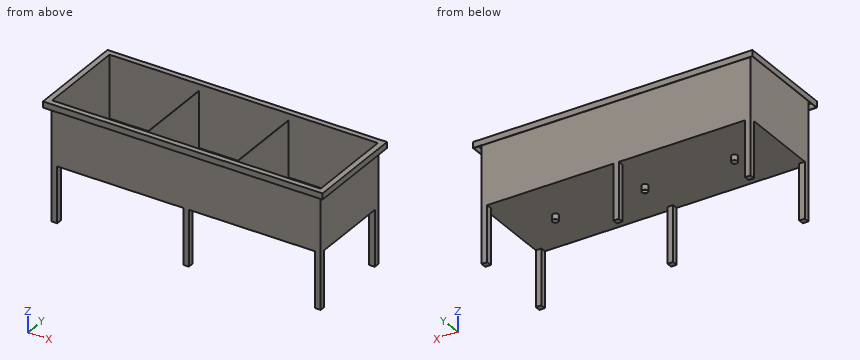
from build123d import *

# Parameters (mm, degrees)
F0_W      = 2412
F0_H      = 806
F1_DEPTH  = 563
F2_T      = -3
F3_W      = 3
F3_H      = 800
F4_DEPTH  = 500
F5_W      = 2506
F5_H      = 900
F5_W_2    = 2412
F5_H_2    = 806
F6_DEPTH  = 4
F7_R      = 25
F8_DEPTH  = 25
F9_R      = 27
F9_R_2    = 25
F10_DEPTH = 50
F11_W     = 2506
F11_H     = 900
F11_W_2   = 2500
F11_H_2   = 894
F12_DEPTH = 50
F13_W     = 50
F13_H     = 50
F14_DEPTH = 500


with BuildPart() as f1:
    # F0 (on Top) → F1 (new body)
    with BuildSketch(Plane.XY):
        with Locations((-1206, -403)):
            Rectangle(F0_W, F0_H)
    extrude(amount=-F1_DEPTH)

    # F2
    f2_openings = [f1.faces().sort_by_distance(p)[0] for p in [
        (-1206, -403, 0),
    ]]
    offset(amount=F2_T, openings=f2_openings)

    # F3 (on face) → F4 (join)
    with BuildSketch(Plane.XY.offset(-560)):
        with Locations((-1607.5, -403)):
            Rectangle(F3_W, F3_H)
        with Locations((-804.5, -403)):
            Rectangle(F3_W, F3_H)
    extrude(amount=F4_DEPTH)

    # F5 (on face) → F6 (join)
    with BuildSketch(Plane.XY):
        with Locations((-1206, -403)):
            Rectangle(F5_W, F5_H)
        with Locations((-1206, -403)):
            Rectangle(F5_W_2, F5_H_2, mode=Mode.SUBTRACT)
    extrude(amount=-F6_DEPTH)

    # F7 (on face) → F8 (cut)
    with BuildSketch(Plane.XY.offset(-560)):
        with Locations((-2009, -403)):
            Circle(F7_R)
        with Locations((-1206, -403)):
            Circle(F7_R)
        with Locations((-403, -403)):
            Circle(F7_R)
    extrude(amount=-F8_DEPTH, mode=Mode.SUBTRACT)

    # F9 (on face) → F10 (join)
    with BuildSketch(Plane(origin=(0, 0, -563), x_dir=(1, 0, 0), z_dir=(0, 0, -1))):
        with Locations((-1206, 403)):
            Circle(F9_R)
        with Locations((-1206, 403)):
            Circle(F9_R_2, mode=Mode.SUBTRACT)
        with Locations((-2009, 403)):
            Circle(F9_R)
        with Locations((-2009, 403)):
            Circle(F9_R_2, mode=Mode.SUBTRACT)
        with Locations((-403, 403)):
            Circle(F9_R)
        with Locations((-403, 403)):
            Circle(F9_R_2, mode=Mode.SUBTRACT)
    extrude(amount=F10_DEPTH)

    # F11 (on face) → F12 (join)
    with BuildSketch(Plane(origin=(0, 0, -4), x_dir=(1, 0, 0), z_dir=(0, 0, -1))):
        with Locations((-1206, 403)):
            Rectangle(F11_W, F11_H)
        with Locations((-1206, 403)):
            Rectangle(F11_W_2, F11_H_2, mode=Mode.SUBTRACT)
    extrude(amount=F12_DEPTH)

    # F13 (on face) → F14 (join)
    with BuildSketch(Plane(origin=(0, 0, -563), x_dir=(1, 0, 0), z_dir=(0, 0, -1))):
        with Locations((-2387, 781)):
            Rectangle(F13_W, F13_H)
        with Locations((-2387, 25)):
            Rectangle(F13_W, F13_H)
        with Locations((-25, 781)):
            Rectangle(F13_W, F13_H)
        with Locations((-25, 25)):
            Rectangle(F13_W, F13_H)
        with Locations((-1206, 781)):
            Rectangle(F13_W, F13_H)
        with Locations((-1206, 25)):
            Rectangle(F13_W, F13_H)
    extrude(amount=F14_DEPTH)


solid = f1.part
Verification items for the finished model (mm, model axes). Give positions to 0.01 mm unless a question says otherwise; leave off trailing zeros. Order: outer loops, then holes, each group sorted by start corner. A loop starts at its lowest first (then second) coordinate and runs counter-clockwise, first axis right, second up. Notation, with made-up numbers: M -28,41 L -23,41 A32 ccw -23,67 Z; hole C 12,82 d5. An arc over 180 degrees is marked long. Answer as a JSON object with one key per item and string values. Group by question number.
1) Cross-section at D-D (x = -611). Enter the section's corners in (y, z), then the cut area to 3 significant figures.
2) Cross-section at A-A (x = -2009). Enter the section's corners in (y, z).
3) Cross-section at B-B (z = -742). Enter the section's corners in (x, y), then the cut area to 3 significant figures.
4) Cross-section at C-C (y = -180.5). Enter the section's corners in (x, z).
5) Scan lines: line 1 along Y through (x, z) = (-1206, -598); line 2 along X through (y, z) = (-475.5, -450.5); line 3 along X through (y, z) = (-403, -595.5). Record each from-to range of solid material in increasing order. Write a range as [from, to].
6) Depth check by flat-ended pin: pin 1 Ø8 at (x, z) = (-1311, -336) entering from +Y; pin 2 Ø25 at (y, z) = (-774.5, -838.5) entering from -X; pin 3 Ø3 at (y, z) = (-69, -460) entering from +X. Enter the tip coordinate at first touch or a pass-through.
Result sheet:
{
 "1": {"outline": "M -853,-54 L -850,-54 L -850,-4 L -806,-4 L -806,-563 L 0,-563 L 0,-4 L 44,-4 L 44,-54 L 47,-54 L 47,0 L -3,0 L -3,-560 L -803,-560 L -803,0 L -853,0 Z", "area": "6,450 mm2"},
 "2": {"outline": "M -853,-54 L -850,-54 L -850,-4 L -806,-4 L -806,-563 L -430,-563 L -430,-613 L -428,-613 L -428,-560 L -803,-560 L -803,0 L -853,0 Z; M -378,-613 L -376,-613 L -376,-563 L 0,-563 L 0,-4 L 44,-4 L 44,-54 L 47,-54 L 47,0 L -3,0 L -3,-560 L -378,-560 Z"},
 "3": {"outline": "M -2412,-806 L -2362,-806 L -2362,-756 L -2412,-756 Z; M -2412,-50 L -2362,-50 L -2362,0 L -2412,0 Z; M -1231,-806 L -1181,-806 L -1181,-756 L -1231,-756 Z; M -1231,-50 L -1181,-50 L -1181,0 L -1231,0 Z; M -50,-806 L 0,-806 L 0,-756 L -50,-756 Z; M -50,-50 L 0,-50 L 0,0 L -50,0 Z", "area": "15,000 mm2"},
 "4": {"outline": "M -2459,-54 L -2456,-54 L -2456,-4 L -2412,-4 L -2412,-563 L 0,-563 L 0,-4 L 44,-4 L 44,-54 L 47,-54 L 47,0 L -3,0 L -3,-560 L -803,-560 L -803,-60 L -806,-60 L -806,-560 L -1606,-560 L -1606,-60 L -1609,-60 L -1609,-560 L -2409,-560 L -2409,0 L -2459,0 Z"},
 "5": {"line 1": "y = [-806, -756], [-430, -428], [-378, -376], [-50, 0]", "line 2": "x = [-2412, -2409], [-1609, -1606], [-806, -803], [-3, 0]", "line 3": "x = [-2036, -2034], [-1984, -1982], [-1233, -1231], [-1181, -1179], [-430, -428], [-378, -376]"},
 "6": {"pin 1": "stops at y = 0", "pin 2": "stops at x = -2412", "pin 3": "stops at x = 0"}
}
